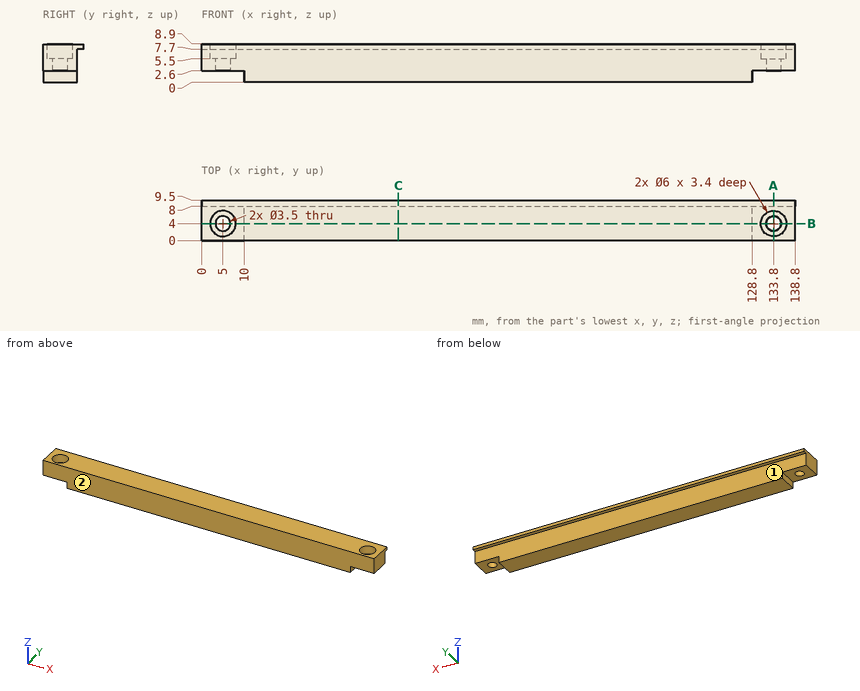
Input: dimensioned drawing with shaded views. Units: mm. Origin: part minimum x, y, z. A direction names the side the tool comes from. Give positions to 0.01 mm unless a question says otherwise; leave off trailing zeros. Write each loop counter-clockwise with the first axis right and the second up, starting at its lowest first coordinate (ties: lowest second). Pieces come first, ordered by that corner, then holes. Notation, with made-up numbers: M -39.75,-18.5 L -4.75,-18.5 A26 ccw -4.75,8.5 Z; hole C 43,68 d4. An arc over 180 degrees is marked long. Write item = value, one per line. Start each with the question number.
1) Cut plane C-C on x = 46. Return the cut outline in (y, z).
2) Material intervals for line 1 along X through (y, z) = (5.75, 6.5); line 2 along Y through (x, z) = (133.8, 3.45); line 3 along Y through (x, z) = (5, 6.75), sorted ascending. Write a range as [from, to].
3) Cut plane A-A on x = 133.8. Return the cut outline in (y, z), then the cut area to 4 significant figures.
4) Reachability of the marked faces 1 and 2 from +Z, -Z, +X, -X, +Y, -Y: full face, straight path, thin tool, end or side. Return the list, or none.
5) Cut plane B-B on y = 4. Return the cut outline in (x, z), then the cut area to 3 significant figures.
6) First-contact query: pin 1 Ø4 at (x, y) = (131.5, 4) entering from -Z; pin 2 Ø1 at (y, z) = (6.5, 2) entering from +X; pin 3 Ø0.8 at (x, y) = (100.5, 9) entering from -Z; pin 4 Ø4 at (x, z) = (82.5, 3) entering from -Y. Flat tips, straight axial feed; report the tip coordinate or a pass-through.
Solved:
q1.outline = M 0,0 L 8,0 L 8,7.7 L 9.5,7.7 L 9.5,8.9 L 0,8.9 Z
q2.line_1 = [0, 2.56], [7.44, 131.36], [136.24, 138.8]
q2.line_2 = [0, 2.25], [5.75, 8]
q2.line_3 = [0, 1], [7, 8]
q3.outline = M 0,2.6 L 2.25,2.6 L 2.25,5.5 L 1,5.5 L 1,8.9 L 0,8.9 Z; M 5.75,2.6 L 8,2.6 L 8,7.7 L 9.5,7.7 L 9.5,8.9 L 7,8.9 L 7,5.5 L 5.75,5.5 Z
q3.area = 21.65 mm2
q4.face_1 = -Z, +X, -X, +Y
q4.face_2 = +Z, -Z, +X, -X, -Y
q5.outline = M 0,2.6 L 3.25,2.6 L 3.25,5.5 L 2,5.5 L 2,8.9 L 0,8.9 Z; M 6.75,2.6 L 10,2.6 L 10,0 L 128.8,0 L 128.8,2.6 L 132.05,2.6 L 132.05,5.5 L 130.8,5.5 L 130.8,8.9 L 8,8.9 L 8,5.5 L 6.75,5.5 Z; M 135.55,2.6 L 138.8,2.6 L 138.8,8.9 L 136.8,8.9 L 136.8,5.5 L 135.55,5.5 Z
q5.area = 1,120 mm2
q6.pin_1 = 2.6
q6.pin_2 = 128.8
q6.pin_3 = 7.7
q6.pin_4 = 0
